Check sheet for the modelled part. Datum: model origin and axes. Units: mm. A direction names the side the tool comes from. Give positions to 0.01 mm unless a question says otherwise; leave off trailing zeros. Loops run counter-clockwise (first coordinate to the right, second up) from the corner with the lowest first, then second, coordinate; pieces in that order, holes last. Notation, with made-up numbers: (79, -19) -> (132, -19) arc R14 ccw to (132, -5) -> close; hole circle Ø7 at (-17, 14.25). An arc over 180 degrees is marked (long way). Write each question's results on one line, items separated by ' | '. Start each with the question number.
Item 1: Cross-section at A-A on z = -2. Enter the section's corners in (x, y).
Item 2: Gauge pin test, flat ends, axial feed: pin 1 Ø3 at (x, y) = (-8.5, 3) entering from +Z; pin 2 Ø1 at (y, z) = (-1, -8.5) entering from +X; pin 3 Ø4 at (y, z) = (1.5, -16) entering from -X (3 decimals); pin 4 Ø3.5 at (x, z) = (0, -12) entering from +Y. Record the tip position at first contact, or that the pin passes through.
Item 3: Cross-section at D-D on x = -34. Enter the section's corners in (y, z), then the cut area to 3 significant figures.
Item 4: Scan lines: line 1 along Z through (x, y) = (0, 2.8); line 2 along Y through (x, z) = (-34, -2.25); line 3 along X through (y, z) = (-2.75, -13). Record each from-to range of solid material in increasing order.
Item 5: Mould release check, pull along Y, two halves, no side actions. Record for faces 1 (the face through (0.1, 2, -9.7)), 2 (the face through (-6, 3, -9)), 3 (the face through (-11, 5, -4)): pulls with the +Y half, pulls with the -Y half, needs draft (parallel to the pull), parting line crosses it, or undercut.
Item 6: Cross-section at C-C on y = 3.5. State how many separate pieces and enclosed holes the cut face has, then the cut area to 3 significant figures.
Item 7: Access from +Z, -Z, +X, -X, +Y, -Y to the whole of each face (thin tool, end or side, straight path). Record for faces 4 (the face through (-39, 0, -4)), 5 (the face through (0.1, -2, -9.5)), 6 (the face through (-33, -1, -9.5)).
Item 8: Cross-section at B-B on y = 0. Enter the section's corners in (x, z).
Autodesk Inventor part; units mm, degrees
ref_plane "YZ Plane" through (0, 0, 0) normal (1, 0, 0) x (0, 1, 0)
ref_plane "XZ Plane" through (0, 0, 0) normal (0, 1, 0) x (-1, 0, 0)
ref_plane "XY Plane" through (0, 0, 0) normal (0, 0, 1) x (1, 0, 0)
sketch "Sketch1" plane through (0, 0, 0) normal (0, 1, 0) x (-1, 0, 0)
  circle A0 centre (0, 0) radius 3 construction
  line L0 (-6, 6) -> (6, 6)
  line L1 (6, 6) -> (39, 0.5)
  line L2 (39, 0.5) -> (39, -9.5)
  line L3 (39, -9.5) -> (29, -9.5)
  line L4 (-6, -19) -> (-6, 6)
  circle A1 centre (0, -13) radius 3 construction
  line L5 (29, -9.5) -> (29, -6)
  line L6 (29, -6) -> (6, -6)
  line L7 (6, -6) -> (6, -19)
  line L8 (6, -19) -> (-6, -19)
  dimension "d0" = 6
  dimension "d1" = 6
  dimension "d2" = 13
  dimension "d4" = 6
  dimension "d5" = 9.5
  dimension "d6" = 45
  dimension "d8" = 6
  dimension "d9" = 10
  dimension "d10" = 12
  dimension "d36" = 12
  dimension "d37" = 6
  dimension "d38" = 13
  dimension "d39" = 10
extrude "Extrusion1" add sketch "Sketch1" along normal mid plane 10
sketch "Sketch2" plane through (0, 5, 0) normal (0, 1, 0) x (1, 0, 0)
  circle A0 centre (0, 0) radius 3
  circle A1 centre (0, 13) radius 3
  dimension "d13" = 6
  dimension "d14" = 13
hole "Hole1" at (0, 5, 0) at (0, 5, -13) direction (0, -1, 0) diameter 6 end through all
sketch "Sketch3" plane through (6, -5, -19) normal (1, 0, 0) x (0, 0, -1)
  line L0 (0, 0) -> (0, 10)
  line L1 (0, 7) -> (-13, 7)
  line L2 (-13, 7) -> (-13, 3)
  line L3 (-13, 3) -> (0, 3)
  line L4 (0, 3) -> (0, 7)
  point P0 (-19, 5)
  point P1 (0, 3)
  dimension "d22" = 13
  dimension "d23" = 4
  dimension "d24" = 2
extrude "Extrusion2" cut sketch "Sketch3" against normal blind 12
sketch "Sketch4" plane through (-29, 5, -9.5) normal (0, 0, -1) x (-1, 0, 0)
  circle A0 centre (5, -5) radius 1.5
  line L0 (10, 0) -> (10, -10)
  point P0 (-29, -5)
  dimension "d27" = 3
  dimension "d28" = 5
hole "Hole2" at (-34, 0, -9.5) direction (0, 0, 1) diameter 2.459 end through all
fillet "Fillet1" radius 6 5 edges at (6, 0, 6) (6, 3.5, -19) (-6, 3.5, -19) (6, -3.5, -19) (-6, -3.5, -19)
equation "\"d15\" = d13"
properties part number "Gripper_Arm_Base" material "Aluminum 6061"
Answer sheet:
1) outline: (-39, -5) -> (-2.24, -5) -> (-2.24, 5) -> (-39, 5) -> close; (2.24, -5) -> (6, -5) -> (6, 5) -> (2.24, 5) -> close; hole circle Ø2.46 at (-34, 0)
2) pin 1: stops at z = 5.83 | pin 2: stops at x = -29 | pin 3: stops at x = -5.905 | pin 4: passes through
3) outline: (-5, -9.5) -> (-1.23, -9.5) -> (-1.23, 1.33) -> (-5, 1.33) -> close; (1.23, -9.5) -> (5, -9.5) -> (5, 1.33) -> (1.23, 1.33) -> close | area: 81.7 mm²
4) line 1: z = -19 to -16, -10 to -3, 3 to 6 | line 2: y = -5 to -1.23, 1.23 to 5 | line 3: x = -6 to -3, 3 to 6
5) face 1: undercut | face 2: needs draft | face 3: pulls with the +Y half
6) separate pieces: 1 | enclosed holes: 2 | area: 561 mm²
7) face 4: +Z, -Z, -X, +Y, -Y | face 5: -Z, +X | face 6: -Z, -X, +Y, -Y
8) outline: (-39, -9.5) -> (-35.23, -9.5) -> (-35.23, 1.13) -> (-39, 0.5) -> close; (-32.77, -9.5) -> (-29, -9.5) -> (-29, -6) -> (6, -6) -> (6, 0) arc R6 ccw to (0, 6) -> (-6, 6) -> (-32.77, 1.54) -> close; hole circle Ø6 at (0, 0)
